Could you check a few things on this model? Use its own coordinates, in mm. A direction names the side the tool comes from. Give positions to 0.01 mm unless a question says otherwise; leave off trailing zeros. Write each loop counter-clockwise with the first axis right and the second up, starting at its lowest first coordinate (ties: lowest second). Pieces come first, ordered by that corner, then holes. Notation, with made-up numbers: M 13.25,39 L 28.25,39 A22 cw 28.25,69 Z; hole C -23,59 d8. An arc over 180 degrees is marked long. Use one line per item in the form item = value.
from build123d import *

# Parameters (mm, degrees)
SKETCH1_W                 = 53
SKETCH1_H                 = 21
BOSS_EXTRUDE1_DEPTH       = 1.6
BOSS_EXTRUDE2_DEPTH       = 0.4
BOSS_EXTRUDE2_DEPTH_BACK  = 7.6
SKETCH3_W                 = 4.2
SKETCH3_H                 = 3.4
BOSS_EXTRUDE3_DEPTH       = 1.7
BOSS_EXTRUDE4_DEPTH       = 0.5
SKETCH_PATTERN1_START     = 1.6
SKETCH_PATTERN1_OUTLINE_W = 4.2
SKETCH_PATTERN1_OUTLINE_H = 3.4
SKETCH_PATTERN1_DEPTH     = 1.7
SKETCH_PATTERN1_START_2   = 3.3
SKETCH_PATTERN1_2_DEPTH   = 0.5
SKETCH6_R                 = 0.6
CUT_EXTRUDE1_DEPTH        = 30.053399113
LPATTERN1_COUNT           = 20
LPATTERN1_PITCH           = 2.65128085
BOSS_EXTRUDE5_DEPTH       = 0.5
SKETCH8_R                 = 0.6
CUT_EXTRUDE2_DEPTH        = 30.053399113
LPATTERN2_COUNT           = 4
LPATTERN2_PITCH           = 2.65128085


# Read off the part's stored shape, not the designer's step: Sketch-Pattern1
with BuildPart() as part:
    # Sketch1 → Boss-Extrude1 (new body)
    with BuildSketch(Plane(origin=(0, 0, 0), x_dir=(1, 0, 0), z_dir=(0, 1, 0))):
        Rectangle(SKETCH1_W, SKETCH1_H)
    extrude(amount=BOSS_EXTRUDE1_DEPTH)

    # Sketch2 → Boss-Extrude2 (add, two sides: drawn at the far end of the back side and taken through both)
    with BuildSketch(Plane.ZY.offset(26.5).offset(-BOSS_EXTRUDE2_DEPTH_BACK)):
        with BuildLine():
            Line((-2.9, 4.8), (2.9, 4.8))
            ThreePointArc((2.9, 4.8), (4.5, 3.2), (2.9, 1.6))
            Line((2.9, 1.6), (-2.9, 1.6))
            ThreePointArc((-2.9, 1.6), (-4.5, 3.2), (-2.9, 4.8))
        make_face()
    extrude(amount=BOSS_EXTRUDE2_DEPTH + BOSS_EXTRUDE2_DEPTH_BACK)

    # Sketch3 → Boss-Extrude3 (add)
    with BuildSketch(Plane(origin=(0, 1.6, 0), x_dir=(1, 0, 0), z_dir=(0, 1, 0))):
        with Locations((15.1, -2.2)):
            Rectangle(SKETCH3_W, SKETCH3_H)
    extrude(amount=BOSS_EXTRUDE3_DEPTH)

    # Sketch4 → Boss-Extrude4 (add)
    with BuildSketch(Plane(origin=(0, 3.3, 0), x_dir=(1, 0, 0), z_dir=(0, 1, 0))):
        with BuildLine():
            Line((14.3, -1.234969734), (15.9, -1.234969734))
            ThreePointArc((15.9, -1.234969734), (16.865030266, -2.2), (15.9, -3.165030266))
            Line((15.9, -3.165030266), (14.3, -3.165030266))
            ThreePointArc((14.3, -3.165030266), (13.334969734, -2.2), (14.3, -1.234969734))
        make_face()
    extrude(amount=BOSS_EXTRUDE4_DEPTH)

    # Sketch-Pattern1 outline → Sketch-Pattern1 (add)
    with BuildSketch(Plane(origin=(0, 0, 0), x_dir=(1, 0, 0), z_dir=(0, 1, 0)).offset(SKETCH_PATTERN1_START)):
        with Locations((-11, -2.2)):
            Rectangle(SKETCH_PATTERN1_OUTLINE_W, SKETCH_PATTERN1_OUTLINE_H)
        with Locations((-11, 3)):
            Rectangle(SKETCH_PATTERN1_OUTLINE_W, SKETCH_PATTERN1_OUTLINE_H)
    extrude(amount=SKETCH_PATTERN1_DEPTH)

    # Sketch-Pattern1 2 outline → Sketch-Pattern1 2 (add)
    with BuildSketch(Plane(origin=(0, 0, 0), x_dir=(1, 0, 0), z_dir=(0, 1, 0)).offset(SKETCH_PATTERN1_START_2)):
        with BuildLine():
            Line((-11.8, -3.165030266), (-10.2, -3.165030266))
            ThreePointArc((-10.2, -3.165030266), (-9.234969734, -2.2), (-10.2, -1.234969734))
            Line((-10.2, -1.234969734), (-11.8, -1.234969734))
            ThreePointArc((-11.8, -1.234969734), (-12.765030266, -2.2), (-11.8, -3.165030266))
        make_face()
        with BuildLine():
            ThreePointArc((-11.8, 3.965030266), (-12.765030266, 3), (-11.8, 2.034969734))
            Line((-11.8, 2.034969734), (-10.2, 2.034969734))
            ThreePointArc((-10.2, 2.034969734), (-9.234969734, 3), (-10.2, 3.965030266))
            Line((-10.2, 3.965030266), (-11.8, 3.965030266))
        make_face()
    extrude(amount=SKETCH_PATTERN1_2_DEPTH)

    # Sketch6 → Cut-Extrude1 (cut, through all)
    with BuildSketch(Plane(origin=(0, 1.6, 0), x_dir=(1, 0, 0), z_dir=(0, 1, 0))):
        with Locations(Location((-25.374336146, 8.615861733, 0), (0, 0, 270))):
            Circle(SKETCH6_R)
        with Locations(Location((-25.374336146, -8.615861733, 0), (0, 0, 90))):
            Circle(SKETCH6_R)
    cut_extrude1 = extrude(amount=-CUT_EXTRUDE1_DEPTH, mode=Mode.SUBTRACT)

    # LPattern1: Cut-Extrude1 ×20
    with Locations(*[(i * LPATTERN1_PITCH, 0, 0) for i in range(1, LPATTERN1_COUNT)]):
        add(cut_extrude1, mode=Mode.SUBTRACT)

    # Sketch7 → Boss-Extrude5 (add)
    with BuildSketch(Plane(origin=(0, 1.6, 0), x_dir=(1, 0, 0), z_dir=(0, 1, 0))):
        Polygon((-5.374011537, 0), (0, 5.374011537), (5.374011537, 0), (0, -5.374011537), align=None)
    extrude(amount=BOSS_EXTRUDE5_DEPTH)

    # Sketch8 → Cut-Extrude2 (cut, through all)
    with BuildSketch(Plane(origin=(0, 1.6, 0), x_dir=(1, 0, 0), z_dir=(0, 1, 0))):
        with Locations(Location((21, 4.25, 0), (0, 0, 270))):
            Circle(SKETCH8_R)
    cut_extrude2 = extrude(amount=-CUT_EXTRUDE2_DEPTH, mode=Mode.SUBTRACT)

    # LPattern2: Cut-Extrude2 ×4
    with Locations(*[(0, 0, i * LPATTERN2_PITCH) for i in range(1, LPATTERN2_COUNT)]):
        add(cut_extrude2, mode=Mode.SUBTRACT)


solid = part.part
1) For faces 1 (the cylindrical face through (-9.235, 3.546, 2.221)), 2 (the flat face through (13, 2, 2)), 3 (the flat face through (-11, 3.8, 2)), 4 (the flat face through (-2.725, 1.846, -2.649)), 5 (the flat face through (2.649, 1.846, -2.725)), which set-ups out of +Z, -Z, +X, -X, +Y, -Y let a thin tool reach every point of the face, with its end or its side?
Checked values:
face_1 = +Y
face_2 = +Z, -Z, +Y
face_3 = +Z, -Z, +X, +Y
face_4 = -Z, +Y
face_5 = -Z, +X, +Y
2) I want a section at B-B, the plane z = 2.2. Please give me the cut outline in (x, y).
Checked values:
outline = M -26.9,1.6 L -26.5,1.6 L -26.5,0 L 26.5,0 L 26.5,1.6 L 17.2,1.6 L 17.2,3.3 L 16.87,3.3 L 16.87,3.8 L 13.33,3.8 L 13.33,3.3 L 13,3.3 L 13,1.6 L 3.17,1.6 L 3.17,2.1 L -3.17,2.1 L -3.17,1.6 L -8.9,1.6 L -8.9,3.3 L -9.23,3.3 L -9.23,3.8 L -12.77,3.8 L -12.77,3.3 L -13.1,3.3 L -13.1,1.6 L -18.9,1.6 L -18.9,4.8 L -26.9,4.8 Z
3) For pin 1 Ø1.6 at (x, z) = (-9.47, 8.62) entering from +Y; pin 2 Ø0.6 at (x, y) = (15, 3.5) entering from +Z; pin 3 Ø6 at (x, z) = (-6, -5) entering from +Y, each with a flat end and sliding along its axis, tell me the tip position at first contact or that it passes through.
Checked values:
pin_1 = 1.6
pin_2 = 3.9
pin_3 = 3.3
4) Thinking about a two-plate mould opening in X: for faces 6 (the flat face through (15, 2, 3.9)), 7 (the cylindrical face through (-12.713, 0.811, 8.694)), 8 (the flat face through (-13.1, 2, -3)), 9 (the flat face through (-26.9, 3, 0)), which applies, released by +X, released by -X, zero draft, split by the parting line, or undercut?
Checked values:
face_6 = zero draft
face_7 = undercut
face_8 = undercut
face_9 = released by -X
5) I want a section at A-A, the plane x = 25. Please give me the cut outline in (y, z).
Checked values:
outline = M 0,-10.5 L 1.6,-10.5 L 1.6,-9.22 L 0,-9.22 Z; M 0,-8.02 L 1.6,-8.02 L 1.6,8.02 L 0,8.02 Z; M 0,9.22 L 1.6,9.22 L 1.6,10.5 L 0,10.5 Z
6) I want a section at C-C, the plane y = 0.9. Count the separate pieces of the cut face and the enclosed holes in it, plus the area to 3 significant figures.
Checked values:
separate_pieces = 1
enclosed_holes = 44
area = 1,060 mm2
7) If I drill on L1, parallel to Z at x = -1.5, y = 0.5; L2, parallel to X at y = 2.8, z = -2.5; L3, parallel to X at y = 1.3, z = -6.5, over which ranges is the centre line in solid material (lowest first)?
Checked values:
L1 = -10.5 to -9.22, -8.02 to 8.02, 9.22 to 10.5
L2 = -26.9 to -18.9, -13.1 to -8.9
L3 = -26.5 to 26.5
